Here's how the part is built. I have some questions about the finished solid (model axes, mm). Face numbers are marked on the shaded views. A direction names the side the tool comes from. Give positions to 0.01 mm unless a question says otherwise; leave off trailing zeros. Loops run counter-clockwise (first coordinate to the right, second up) from the corner with the lowest first, then second, coordinate; pieces in that order, holes last. Notation, with made-up numbers: (-11.5, 86) - (24.5, 86) arc R30 cw to (24.5, 118) - close; hole circle Ø11 at (42, 82.5). An arc over 180 degrees is marked (long way). Use one line per item in the form item = value.
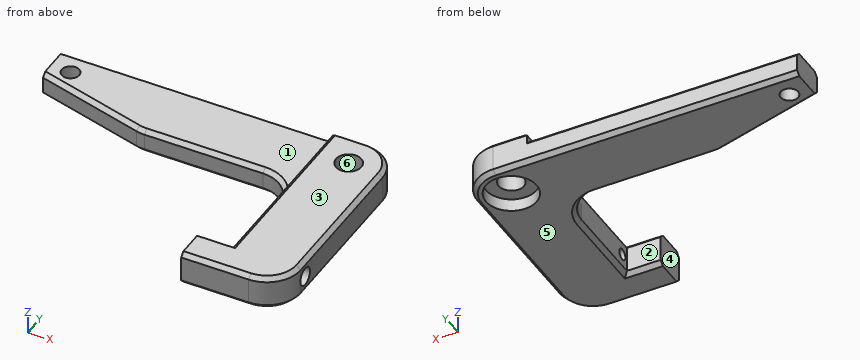
from build123d import *

# Parameters (mm, degrees)
BASE_EXTRUDE_DEPTH = 12.7
SKETCH2_R          = 4.7625
CUT_EXTRUDE1_DEPTH = 135.554087638
SKETCH3_R          = 3.302
CUT_EXTRUDE2_DEPTH = 106.159296474
CHAMFER1_SIZE      = 11.43
CHAMFER1_SIZE2     = 42.657340731
SKETCH5_W          = 101.6
SKETCH5_H          = 25.4
CUT_EXTRUDE4_DEPTH = 3.429
FILLET2_R          = 12.7
CHAMFER2_SIZE      = 1.5875
CHAMFER3_SIZE      = 1.5875
SKETCH8_R          = 9.525
CUT_EXTRUDE5_DEPTH = 4.7752


with BuildPart() as part:
    # Sketch1 → Base-Extrude (new body)
    with BuildSketch(Plane.XY):
        Polygon((-114.3, 12.7), (-114.3, -12.7), (-12.7, -12.7), (-12.7, -57.15), (-25.4, -57.15), (-25.4, -69.85), (12.7, -69.85), (12.7, 12.7), align=None)
    extrude(amount=BASE_EXTRUDE_DEPTH)

    # Sketch2 → Cut-Extrude1 (cut, through all)
    with BuildSketch(Plane.XY.offset(12.7)):
        Circle(SKETCH2_R)
    extrude(amount=-CUT_EXTRUDE1_DEPTH, mode=Mode.SUBTRACT)

    # Sketch3 → Cut-Extrude2 (cut, through all)
    with BuildSketch(Plane(origin=(-40.826123223, 4.303739396, 12.7), x_dir=(1, 0, 0), z_dir=(0, 0, 1))):
        with Locations((-65.853876777, -0.493739396)):
            Circle(SKETCH3_R)
    extrude(amount=-CUT_EXTRUDE2_DEPTH, mode=Mode.SUBTRACT)

    # Chamfer1
    chamfer1_edges = [part.edges().sort_by_distance(p)[0] for p in [
        (-114.3, -12.7, 6.35),
    ]]
    chamfer1_side = [part.faces().sort_by_distance(p)[0] for p in [
        (-114.3, 0, 6.35),
    ]]
    chamfer(chamfer1_edges, length=CHAMFER1_SIZE, length2=CHAMFER1_SIZE2, reference=chamfer1_side[0])

    # Sketch5 → Cut-Extrude4 (cut)
    with BuildSketch(Plane(origin=(-65.557986772, -0.200650606, 12.7), x_dir=(1, 0, 0), z_dir=(0, 0, 1))):
        with Locations((2.057986772, 0.200650606)):
            Rectangle(SKETCH5_W, SKETCH5_H)
    extrude(amount=-CUT_EXTRUDE4_DEPTH, mode=Mode.SUBTRACT)

    # Sketch7 → Hole1 (revolve, cut)
    with BuildSketch(Plane(origin=(12.7, -53.975, 6.35), x_dir=(0, 0, -1), z_dir=(0, 1, 0))):
        Polygon((0, 0), (0, 127), (2.108198174, 127), (2.108198174, 126.997460002), (2.108198174, 12.699989143), (2.740657626, 12.699989), (3.373117078, 12.699989), (3.373117078, 6.3499945), (3.373117078, 0), align=None)
    revolve(axis=Axis((12.7, -53.975, 6.35), (-1, 0, 0)), mode=Mode.SUBTRACT)

    # Fillet2
    # the kernel refuses this fillet: 12.7 mm, written as the material it adds along each edge
    with BuildSketch(Plane(origin=(-12.7, -12.7, 0), x_dir=(-1, 0, 0), z_dir=(0, 0, 1))) as fillet2_piece_1:
        with BuildLine():
            CenterArc((FILLET2_R, FILLET2_R), FILLET2_R, 180, 90)
            Line((0, FILLET2_R), (0, 0))
            Line((0, 0), (FILLET2_R, 0))
        make_face()
    extrude(amount=9.271)
    # the kernel refuses this fillet: 12.7 mm, written as the material it takes off along each edge
    with BuildSketch(Plane(origin=(12.7, 12.7, -31.75), x_dir=(0, -1, 0), z_dir=(0, 0, 1))) as fillet2_2_piece_1:
        with BuildLine():
            CenterArc((FILLET2_R, -FILLET2_R), FILLET2_R, 90, 90)
            Line((0, -FILLET2_R), (0, 0))
            Line((0, 0), (FILLET2_R, 0))
        make_face()
    extrude(amount=76.2, mode=Mode.SUBTRACT)
    with BuildSketch(Plane(origin=(12.7, -69.85, -31.75), x_dir=(0, 1, 0), z_dir=(0, 0, 1))) as fillet2_2_piece_2:
        with BuildLine():
            CenterArc((FILLET2_R, FILLET2_R), FILLET2_R, 180, 90)
            Line((0, FILLET2_R), (0, 0))
            Line((0, 0), (FILLET2_R, 0))
        make_face()
    extrude(amount=76.2, mode=Mode.SUBTRACT)
    with BuildSketch(Plane(origin=(-71.642659269, -12.7, -4.179966798), x_dir=(1, 0, 0), z_dir=(0, 0, 1))) as fillet2_2_piece_3:
        with BuildLine():
            CenterArc((FILLET2_R * 0.131652497587, FILLET2_R), FILLET2_R, 255, 15)
            Line((-FILLET2_R * 0.127166547515, FILLET2_R * 0.0340741737109), (0, 0))
            Line((0, 0), (FILLET2_R * 0.131652497587, 0))
        make_face()
    extrude(amount=17.630933597, mode=Mode.SUBTRACT)

    # Chamfer2
    chamfer2_edges = [part.edges().sort_by_distance(p)[0] for p in [
        (-57.15, 12.7, 0),
        (12.7, -28.575, 0),
        (-12.7, -69.85, 0),
        (8.980256121, -66.130256121, 0),
        (8.980256121, 8.980256121, 0),
    ]]
    chamfer(chamfer2_edges, length=CHAMFER2_SIZE)

    # Chamfer3
    chamfer3_edges = [part.edges().sort_by_distance(p)[0] for p in [
        (-19.05, -57.15, 0),
    ]]
    chamfer(chamfer3_edges, length=CHAMFER3_SIZE)
    chamfer3_2_edges = [part.edges().sort_by_distance(p)[0] for p in [
        (-12.7, -41.275, 0),
        (-16.419743879, -16.419743879, 0),
        (-47.685336275, -12.7, 0),
        (-71.628355191, -12.591349739, 0),
        (-93.778837211, -6.768628997, 0),
    ]]
    chamfer(chamfer3_2_edges, length=CHAMFER3_SIZE)
    chamfer3_3_edges = [part.edges().sort_by_distance(p)[0] for p in [
        (-19.05, -57.15, 12.7),
    ]]
    chamfer(chamfer3_3_edges, length=CHAMFER3_SIZE)
    chamfer3_4_edges = [part.edges().sort_by_distance(p)[0] for p in [
        (-12.7, -22.225, 12.7),
    ]]
    chamfer(chamfer3_4_edges, length=CHAMFER3_SIZE)
    chamfer3_5_edges = [part.edges().sort_by_distance(p)[0] for p in [
        (-16.419743879, -16.419743879, 9.271),
        (-47.685336275, -12.7, 9.271),
        (-71.628355191, -12.591349739, 9.271),
        (-93.778837211, -6.768628997, 9.271),
    ]]
    chamfer(chamfer3_5_edges, length=CHAMFER3_SIZE)
    chamfer3_6_edges = [part.edges().sort_by_distance(p)[0] for p in [
        (-12.7, -69.85, 12.7),
        (8.980256121, 8.980256121, 12.7),
        (12.7, -28.575, 12.7),
        (8.980256121, -66.130256121, 12.7),
        (-5.55625, 12.7, 12.7),
    ]]
    chamfer(chamfer3_6_edges, length=CHAMFER3_SIZE)
    chamfer3_7_edges = [part.edges().sort_by_distance(p)[0] for p in [
        (-63.5, 12.7, 9.271),
    ]]
    chamfer(chamfer3_7_edges, length=CHAMFER3_SIZE)

    # Sketch8 → Cut-Extrude5 (cut)
    with BuildSketch(Plane(origin=(0, 0, 0), x_dir=(-1, 0, 0), z_dir=(0, 0, -1))):
        Circle(SKETCH8_R)
    extrude(amount=-CUT_EXTRUDE5_DEPTH, mode=Mode.SUBTRACT)


solid = part.part
(1) If we section it at C-C (y = -7): List the corners of the cut face in (x, z) for me.
Geometry says:
outline = (-92.92, 1.59) - (-86.78, 0) - (-6.46, 0) - (-6.46, 4.78) - (6.46, 4.78) - (6.46, 0) - (11.11, 0) - (12.7, 1.59) - (12.7, 11.11) - (11.11, 12.7) - (-11.11, 12.7) - (-12.7, 11.11) - (-12.7, 9.27) - (-86.78, 9.27) - (-92.92, 7.68) - close
(2) If we section it at D-D (x = -87): List the corners of the cut face in (y, z) for me, plus the area to 3 significant figures.
Geometry says:
outline = (-8.59, 1.59) - (-6.94, 0) - (11.11, 0) - (12.7, 1.59) - (12.7, 7.68) - (11.11, 9.27) - (-6.94, 9.27) - (-8.59, 7.68) - close
area = 192 mm²
(3) Thinking about a two-plate mould opening in X: for the marked faces 4, 5 and 6, which applies, pulls with the +X half, pulls with the -X half, needs draft (parallel to the pull), parting line crosses it, or undercut?
Geometry says:
face_4 = pulls with the -X half
face_5 = needs draft
face_6 = undercut
(4) For the marked faces 1, 2 and 3, which set-ups out of +Z, -Z, +X, -X, +Y, -Y let a thin tool reach every point of the face, with its end or its side?
Geometry says:
face_1 = +Z, -X, +Y
face_2 = +Z, -Z, -X
face_3 = +Z, +X, -X, +Y, -Y
(5) If we section it at B-B (x = -106.68): List the corners of the cut face in (y, z) for me.
Geometry says:
outline = (-3.31, 1.59) - (-1.67, 0) - (0.51, 0) - (0.51, 9.27) - (-1.67, 9.27) - (-3.31, 7.68) - close; (7.11, 0) - (11.11, 0) - (12.7, 1.59) - (12.7, 7.68) - (11.11, 9.27) - (7.11, 9.27) - close
(6) For P1, Ø12.5, axis at x = 0, y = 0, coming from the -Z side; P2, Ø6.5, axis at y = -63.5, z = 3.5, coming from the -X side; P3, Ø6.5, axis at y = -53.975, z = 6.35, coming from the +X side; P4, Ø5.5, axis at x = -106.68, y = 3.81, coming from the -Z side, each with a flat end and sliding along its axis, tell me the tip position at first contact or that it passes through.
Geometry says:
P1 = 4.78
P2 = -25.4
P3 = 0
P4 = through
(7) If we section it at A-A (x = -55): List the corners of the cut face in (y, z) for me.
Geometry says:
outline = (-12.7, 1.59) - (-11.11, 0) - (11.11, 0) - (12.7, 1.59) - (12.7, 7.68) - (11.11, 9.27) - (-11.11, 9.27) - (-12.7, 7.68) - close
(8) If I drill on probe 1 along Y at (x, z) = (-8, 6.35); probe 2 along Z at (x, y) = (-49, -6.5); probe 3 along X at (y, z) = (-38, 3.25), over which ranges is the centre line in solid material (lowest first)?
Geometry says:
probe_1 = -69.85 to -56.08, -51.87 to 12.7
probe_2 = 0 to 9.27
probe_3 = -12.7 to 12.7
